```python
from build123d import *
from build123d.topology import SkipClean

# Parameters (mm, degrees)
BOSS_EXTRU_1_START      = 70
BOSS_EXTRU_1_DEPTH      = 70
BOSS_EXTRU_2_DEPTH      = 25
ESQUISSE7_R             = 10
ENL_V_MAT_EXTRU_1_DEPTH = 50
CONG_3_R                = 10
ECHELLE1_SCALE          = 0.25


with BuildPart() as part:
    # Esquisse1 → Révolution1 (revolve)
    with BuildSketch(Plane.XY, mode=Mode.PRIVATE) as r_volution1_sk:
        with BuildLine():
            Line((-5, 34.242293075), (-36.242368939, 34.242293075))
            Line((-36.242368939, 34.242293075), (-36.242368939, 39.242293075))
            Line((-36.242368939, 39.242293075), (-38.705375435, 39.242293075))
            Line((-38.705375435, 39.242293075), (-38.705375435, 79.242293075))
            Line((-38.705375435, 79.242293075), (-36.242368939, 79.242293075))
            Line((-36.242368939, 79.242293075), (-36.242368939, 84.242293075))
            Line((-36.242368939, 84.242293075), (-32, 84.242293075))
            Line((-32, 84.242293075), (0, 84.242293075))
            Line((0, 84.242293075), (0, 81.713773078))
            Line((0, 81.713773078), (-32, 81.713773078))
            Line((-32, 81.713773078), (-32, 51.242293075))
            ThreePointArc((-32, 51.242293075), (-31.414213562, 49.828079513), (-30, 49.242293075))
            Line((-30, 49.242293075), (-25, 49.242293075))
            Line((-25, 49.242293075), (-25, 46.233820065))
            Line((-25, 46.233820065), (-5, 46.233820065))
            Line((-5, 46.233820065), (-5, 34.242293075))
        make_face()
    revolve(r_volution1_sk.sketch.rotate(Axis((0, 190.222222222, 0), (0, -1, 0)), 270), axis=Axis((0, 190.222222222, 0), (0, -1, 0)))

    # Esquisse2 → Boss.-Extru.1 (add)
    with SkipClean():  # the faces are left unmerged after this step: merging them gives an invalid solid
        with BuildSketch(Plane(origin=(0, 84.242293075, 0), x_dir=(1, 0, 0), z_dir=(0, 1, 0)).offset(BOSS_EXTRU_1_START)):
            with BuildLine():
                Line((-10, 34.835460472), (-10, -34.835460472))
                ThreePointArc((-10, -34.835460472), (0, -36.242368939), (10, -34.835460472))
                Line((10, -34.835460472), (10, 34.835460472))
                ThreePointArc((10, 34.835460472), (0, 36.242368939), (-10, 34.835460472))
            make_face()
        extrude(amount=-BOSS_EXTRU_1_DEPTH)

    # Esquisse6 → Boss.-Extru.2 (add, symmetric)
    with SkipClean():  # the faces are left unmerged after this step: merging them gives an invalid solid
        with BuildSketch(Plane.ZY):
            with BuildLine():
                ThreePointArc((-34.835460472, 154.242293075), (0, 185.852500498), (34.835460472, 154.242293075))
                ThreePointArc((34.835460472, 154.242293075), (0, 115.852500498), (-34.835460472, 154.242293075))
            make_face()
        extrude(amount=BOSS_EXTRU_2_DEPTH, both=True)

    # Esquisse7 → Enlèv. mat.-Extru.1 (cut)
    with SkipClean():  # the faces are left unmerged after this step: merging them gives an invalid solid
        with BuildSketch(Plane.ZY.offset(25)):
            with Locations((0, 150.852500498)):
                Circle(ESQUISSE7_R)
        extrude(amount=-ENL_V_MAT_EXTRU_1_DEPTH, mode=Mode.SUBTRACT)

    # Congé3
    # the kernel refuses this fillet: 10 mm, written as the material it takes off along each edge
    with BuildSketch(Plane(origin=(10, 172.708919448, 34.835460472), x_dir=(-0.9902475852004595, 0, 0.1393187711855749), z_dir=(0, -1, 0))) as cong_3_piece_1_section:
        with BuildLine():
            CenterArc((8.705296899, 9.902475852), CONG_3_R, 188.0084284, 90)
            Line((-1.197178953, 8.50928814), (0, 0))
            ThreePointArc((0, 0), (5.049242305, -0.353450615), (10.098484611, 0))
        make_face()
    cong_3_piece_1 = extrude(amount=88.466626373, mode=Mode.PRIVATE)
    cong_3_piece_1 = cong_3_piece_1 - Plane(origin=(7.456754733, 150.852500498, 0), x_dir=(0, 0.09685121648897653, -0.9952988706235959), z_dir=(-1, 0, 0)) * Cylinder(35, 218, mode=Mode.PRIVATE)
    add(cong_3_piece_1, mode=Mode.SUBTRACT)
    with BuildSketch(Plane(origin=(10, 172.708919448, -34.835460472), x_dir=(-0.9902475852004589, 0, -0.13931877118558042), z_dir=(0, -1, 0))) as cong_3_piece_2_section:
        with BuildLine():
            CenterArc((8.705296899, -9.902475852), CONG_3_R, 81.9915716, 90)
            Line((-1.197178953, -8.50928814), (0, 0))
            ThreePointArc((0, 0), (5.049242305, 0.353450615), (10.098484611, 0))
        make_face()
    cong_3_piece_2 = extrude(amount=88.466626373, mode=Mode.PRIVATE)
    cong_3_piece_2 = cong_3_piece_2 - Plane(origin=(7.456771832, 150.852500498, 0), x_dir=(0, 0.09685121648897653, -0.9952988706235959), z_dir=(-1, 0, 0)) * Cylinder(35, 218, mode=Mode.PRIVATE)
    add(cong_3_piece_2, mode=Mode.SUBTRACT)
    with BuildSketch(Plane(origin=(-10, 172.708919448, -34.835460472), x_dir=(0.990247585200459, 0, -0.13931877118557906), z_dir=(0, -1, 0))) as cong_3_piece_3_section:
        with BuildLine():
            CenterArc((8.705296899, 9.902475852), CONG_3_R, 188.0084284, 90)
            Line((-1.197178953, 8.50928814), (0, 0))
            ThreePointArc((0, 0), (5.049242305, -0.353450615), (10.098484611, 0))
        make_face()
    cong_3_piece_3 = extrude(amount=88.466626373, mode=Mode.PRIVATE)
    cong_3_piece_3 = cong_3_piece_3 - Plane(origin=(-7.456771832, 150.852500498, 0), x_dir=(0, 0.09685121648897653, -0.9952988706235959), z_dir=(-1, 0, 0)) * Cylinder(35, 218, mode=Mode.PRIVATE)
    add(cong_3_piece_3, mode=Mode.SUBTRACT)
    with BuildSketch(Plane(origin=(-10, 172.708919448, 34.835460472), x_dir=(0.9902475852004595, 0, 0.1393187711855749), z_dir=(0, -1, 0))) as cong_3_piece_4_section:
        with BuildLine():
            CenterArc((8.705296899, -9.902475852), CONG_3_R, 81.9915716, 90)
            Line((-1.197178953, -8.50928814), (0, 0))
            ThreePointArc((0, 0), (5.049242305, 0.353450615), (10.098484611, 0))
        make_face()
    cong_3_piece_4 = extrude(amount=88.466626373, mode=Mode.PRIVATE)
    cong_3_piece_4 = cong_3_piece_4 - Plane(origin=(-7.456754733, 150.852500498, 0), x_dir=(0, 0.09685121648897653, -0.9952988706235959), z_dir=(-1, 0, 0)) * Cylinder(35, 218, mode=Mode.PRIVATE)
    add(cong_3_piece_4, mode=Mode.SUBTRACT)


with BuildPart() as part_1:
    # Echelle1: scaled about (0, 111.005849146, 2.25e-07)
    add(part.part.scale(ECHELLE1_SCALE).moved(Location((0, 83.25438686, 1.69e-07))))


solid = part_1.part
```
Verification items for the finished model (mm, model axes). A direction names the side the tool comes from. Round coordinates to 2 decimals unless told otherwise and drop trailing zeros. Loops run counter-clockwise (first coordinate to the right, second up) from the corner with the lowest first, then second, coordinate; pieces in that order, holes last. Notation, with made-up numbers: (54.25, 42.25) -> (66.25, 42.25) arc R15 cw to (66.25, 71.25) -> close; hole circle Ø4 at (7, 71). An arc over 180 degrees is marked (long way). Answer as a JSON object with one key per item and string values.
Q1. Section check B-B (y = 97). Record the boundary of the cut face in (x, z), then the cut area to 3 significant figures.
Data:
{"outline": "circle Ø19.35 at (0, 0); hole circle Ø16 at (0, 0)", "area": "93.1 mm2"}
Q2. Access from +Z, -Z, +X, -X, +Y, -Y to the whole of each face (thin tool, end or side, straight path). Record for faces 4 (the flat face through (3, 103.065, -9)), 5 (the flat face through (-6.25, 119, -2)), 6 (the cylindrical face through (1.22, 93.29, -0.27)), 7 (the flat face through (2, 91.815, 0)).
Data:
{"face 4": "none", "face 5": "+Z, -Z, -X, +Y", "face 6": "-Y", "face 7": "+Z, -Z, +X, -X, -Y"}
Q3. Draft check along Y on faces 1 (the flat face through (-9, 93.065, -3)), 2 (the flat face through (6.25, 119, -2)), 3 (the cylindrical face through (2.722, 103.699, 8.642)). Enter one of: pulls with the +Y half, pulls with the -Y half, needs draft (parallel to the pull), parting line crosses it, or undercut.
Data:
{"face 1": "pulls with the -Y half", "face 2": "needs draft", "face 3": "undercut"}
Q4. Scan lines: line 1 (X direction, y = 95, z = 0); line 2 (X direction, y = 97, z = -0.25); line 3 (Y direction, x = -5.75, z = -3). Record each from-to range of solid material in increasing order. Write a range as from..to.
Data:
{"line 1": "x = -9.68..-6.25, 6.25..9.68", "line 2": "x = -9.67..-8, 8..9.67", "line 3": "y = 91.81..95.56, 103.68..104.31, 112.75..129.19"}
Q5. Section check A-A (x = 3). State how many separate pieces and enclosed holes the cut face has, then the cut area to 3 significant figures.
Data:
{"separate pieces": "2", "enclosed holes": "2", "area": "319 mm2"}
Q6. Section check C-C (y = 113). Record the boundary of the cut face in (x, z).
Data:
{"outline": "(-6.25, -3.62) -> (-2.5, -3.62) -> (-2.5, -6.56) arc R2.5 ccw to (2.5, -6.56) -> (2.5, -3.62) -> (6.25, -3.62) -> (6.25, 3.62) -> (2.5, 3.62) -> (2.5, 6.56) arc R2.5 ccw to (-2.5, 6.56) -> (-2.5, 3.62) -> (-6.25, 3.62) -> close"}
Q7. Go/stop test with flat-tipped pins: P1, Ø8, axis at x = 0, y = 120.5, coming from the -Z side; P2, Ø3, axis at x = -3.5, y = 124, coming from the -Z side; P3, Ø2, axis at x = -5.5, y = 113.5, coming from the +Z side. Record where each tip stops, or that it passes through.
Data:
{"P1": "stops at z = -9.06", "P2": "stops at z = -8.61", "P3": "stops at z = 5.89"}
